For this review, take the finished solid that the model builds, in its own axes (mm). Face numbers are marked on the shaded views. Give positions to 0.01 mm unless a question says otherwise; leave off trailing zeros. Loops run counter-clockwise (first coordinate to the right, second up) from the corner with the lowest first, then second, coordinate; pieces in that order, holes last.
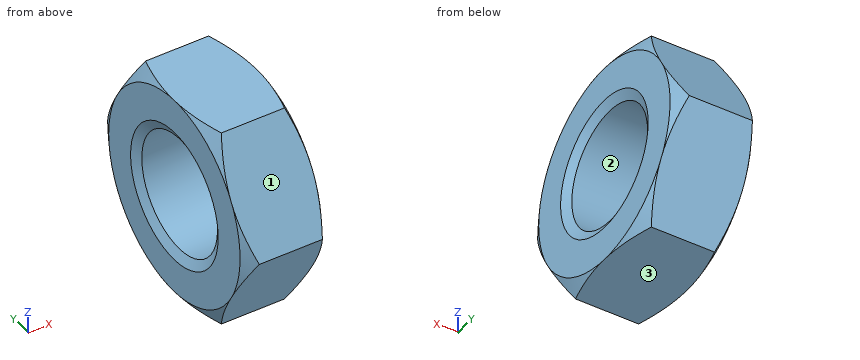
Autodesk Inventor part; units mm, degrees
ref_plane "Work Plane1" through (-35.3709, 0, 0) normal (0, -0.8660254, -0.5) x (1, 0, 0)
ref_plane "YZ Plane" through (0, 0, 0) normal (1, 0, 0) x (0, 1, 0)
ref_plane "XZ Plane" through (0, 0, 0) normal (0, 1, 0) x (-1, 0, 0)
sketch "草圖1" plane through (0, 0, 0) normal (1, 0, 0) x (0, 1, 0)
  line L0 (-17.3205, 0) -> (-8.6603, 15)
  line L1 (-8.6603, 15) -> (8.6603, 15)
  line L2 (8.6603, 15) -> (17.3205, 0)
  line L3 (17.3205, 0) -> (8.6603, -15)
  line L4 (8.6603, -15) -> (-8.6603, -15)
  line L5 (-8.6603, -15) -> (-17.3205, 0)
  point P0 (0, 0)
  point P1 (0, 0)
  dimension "d0" = 34.641
extrude "本體" add sketch "草圖1" along normal blind 12
sketch "草圖2" plane through (0, 0, 0) normal (0, 0, 1) x (1, 0, 0)
  line L0 (0, 8.6603) -> (0, 17.3205)
  line L1 (0, 17.3205) -> (12, 17.3205)
  line L2 (12, 8.6603) -> (12, 17.3205)
  line L3 (-2.4, 0) -> (14.4, 0)
  line L4 (1.3397, 17.3205) -> (0, 15)
  line L5 (10.6603, 17.3205) -> (12, 15)
  dimension "d3" = 30
  dimension "d4" = 30
  dimension "d5" = 30
  dimension "d6" = 30
revolve "倒角1" cut sketch "草圖2" angle 360 about axis through (-10, 0, 0) along (1, 0, 0)
sketch "草圖3" plane through (12, 0, 0) normal (1, 0, 0) x (0, 0, -1)
  arc A0 (-7.5, -12.9904) -> (7.5, -12.9904) centre (0, 0) ccw
hole "螺紋" at (12, 0, 0) direction (-1, 0, 0) diameter 17.294 end through all
chamfer "倒角2" distance 1.3532 angle 30 1 edges at (12, 0, 8.647) measured on face at (12, -12.8065, -0.3474)
chamfer "倒角3" distance 1.3532 angle 30 1 edges at (0, 0, 8.647) measured on face at (0, -12.8065, -0.3474)
ref_plane "Work Plane1" through (-35.3709, 0, 0) normal (0, -0.8660254, -0.5) x (1, 0, 0)
equation "\"d0\" = 1.1547 * SW"
equation "\"d1\" = KOH"
equation "\"d3\" = ANG1"
equation "\"d4\" = ANG2"
equation "\"d5\" = SW0"
equation "\"d6\" = SW01"
equation "\"d8\" = -0.5 * GD1 + 0.5 * NND"
equation "\"d40\" = -0.5 * GD1 + 0.5 * NND"
equation "\"d10\" = -0.5 * GD1 + 0.5 * NND"
equation "\"d41\" = -0.5 * GD1 + 0.5 * NND"
equation "\"ANG1\" = 30deg"
equation "\"ANG2\" = 30deg"
equation "\"KOH\" = 12"
equation "\"SW0\" = SW"
equation "\"SW01\" = SW"
equation "\"GUL\" = 0.541266 * PTC"
equation "\"TOA\" = 30deg"
equation "\"PTC\" = 2.5"
equation "\"E0\" = 1.155 * SW"
equation "\"GAL\" = 0.541266 * PTC"
properties part number "AS 1112 - M20" material "鋼、可鍛"
Item 1: Take a section at A-A on x = 4. Give the boundary of the cut face in (y, z).
Answer:
outline: (-17.32, 0) - (-8.66, -15) - (8.66, -15) - (17.32, 0) - (8.66, 15) - (-8.66, 15) - close; hole circle Ø17.29 at (0, 0)
Item 2: The part is to be moulded in two halves that separate along Y. For the marked faces 1, 2 and 3, say which applies: released by +Y, released by -Y, zero draft, split by the parting line, or undercut.
Answer:
face 1: released by -Y
face 2: undercut
face 3: zero draft
Item 3: Clearance check with flat-ended pins moving along their axes: pin 1 Ø5 at (x, z) = (3, 5) entering from -Y; pin 2 Ø3 at (x, z) = (3.5, -6.5) entering from +Y; pin 3 Ø2 at (x, y) = (2, 13.5) entering from -Z. State where each tip first meets the part, or that it passes through.
Answer:
pin 1: stops at y = -15.88
pin 2: stops at y = 14.43
pin 3: stops at z = -8.35
Item 4: For L1, parallel to Y at x = 6.75, z = 0; L2, parallel to Z at x = 9, y = 0; L3, parallel to Y at x = 8.5, z = -1.25, list the stretches that pass through material, from the lowest coordinate up.
Answer:
L1: y = -17.32 to -8.65, 8.65 to 17.32
L2: z = -15 to -8.65, 8.65 to 15
L3: y = -16.6 to -8.56, 8.56 to 16.6
